```python
from build123d import *

# Parameters (mm, degrees)
F0_R     = 2.5
F1_DEPTH = 7.5
F2_R     = 1
F3_DEPTH = 10
F4_DEPTH = 25


with BuildPart() as f1:
    # F0 (on Top) → F1 (new body)
    with BuildSketch(Plane.XY):
        with BuildLine():
            ThreePointArc((1.4624940646, 33.6666666667), (3.832617517, 34.7501387667), (5.5866740582, 36.6774899598))
            ThreePointArc((5.5866740582, 36.6774899598), (6.2675107251, 38.2771217946), (6.5, 40))
            ThreePointArc((6.5, 40), (-1.7228782054, 46.2675107251), (-5.5866740582, 36.6774899598))
            ThreePointArc((-5.5866740582, 36.6774899598), (-3.832617517, 34.7501387667), (-1.4624940646, 33.6666666667))
            ThreePointArc((-1.4624940646, 33.6666666667), (-0.1677183698, 35.4905940254), (1.5, 34))
            ThreePointArc((1.5, 34), (1.4905940254, 33.8322816302), (1.4624940646, 33.6666666667))
        make_face()
        with Locations((0, 40)):
            Circle(F0_R, mode=Mode.SUBTRACT)
        with BuildLine():
            ThreePointArc((-5.3332565238, 25.44712901), (2.3423382025, 25.8942744974), (9.8131006729, 24.0770233871))
            ThreePointArc((9.8131006729, 24.0770233871), (4.8098794275, 29.40789523), (5.5866740582, 36.6774899598))
            ThreePointArc((5.5866740582, 36.6774899598), (3.832617517, 34.7501387667), (1.4624940646, 33.6666666667))
            ThreePointArc((1.4624940646, 33.6666666667), (0, 32.5), (-1.4624940646, 33.6666666667))
            ThreePointArc((-1.4624940646, 33.6666666667), (-3.832617517, 34.7501387667), (-5.5866740582, 36.6774899598))
            ThreePointArc((-5.5866740582, 36.6774899598), (-4.3898764062, 32.979997265), (-4.9088964418, 29.128452763))
            ThreePointArc((-4.9088964418, 29.128452763), (-4.9503969095, 29.0195498849), (-4.993341291, 28.9112082687))
            Line((-4.993341291, 28.9112082687), (-5.3332565238, 25.44712901))
        make_face()
        with BuildLine():
            ThreePointArc((-10.9419213055, 23.5854692161), (-13.9912480869, -21.9144923959), (26, 0))
            ThreePointArc((26, 0), (21.5770783182, 14.5061949267), (9.8131006729, 24.0770233871))
            ThreePointArc((9.8131006729, 24.0770233871), (2.3423382025, 25.8942744974), (-5.3332565238, 25.44712901))
            Line((-5.3332565238, 25.44712901), (-5.7464520703, 21.2362494006))
            ThreePointArc((-5.7464520703, 21.2362494006), (13.371201413, 17.4702882854), (22, 0))
            ThreePointArc((22, 0), (-10.5068405661, -19.3288980886), (-11.9642092108, 18.4623318668))
            Line((-11.9642092108, 18.4623318668), (-10.9419213055, 23.5854692161))
        make_face()
        with BuildLine():
            ThreePointArc((-9.8131006729, 24.0770233871), (-10.3804210274, 23.837929006), (-10.9419213055, 23.5854692161))
            Line((-10.9419213055, 23.5854692161), (-11.9642092108, 18.4623318668))
            ThreePointArc((-11.9642092108, 18.4623318668), (-9.9487622141, 19.6219807972), (-7.8221766033, 20.5624306245))
            Line((-7.8221766033, 20.5624306245), (-7.3939510007, 24.9264816731))
            ThreePointArc((-7.3939510007, 24.9264816731), (-8.6140032313, 24.5315908235), (-9.8131006729, 24.0770233871))
        make_face()
        with BuildLine():
            ThreePointArc((-7.326121242, 25.6177353666), (-8.504893301, 24.7429137255), (-9.8131006729, 24.0770233871))
            ThreePointArc((-9.8131006729, 24.0770233871), (-8.6140032313, 24.5315908235), (-7.3939510007, 24.9264816731))
            Line((-7.3939510007, 24.9264816731), (-7.326121242, 25.6177353666))
        make_face()
        with BuildLine():
            Line((-9.8358558903, 29.128452763), (-10.9419213055, 23.5854692161))
            ThreePointArc((-10.9419213055, 23.5854692161), (-10.3804210274, 23.837929006), (-9.8131006729, 24.0770233871))
            ThreePointArc((-9.8131006729, 24.0770233871), (-8.504893301, 24.7429137255), (-7.326121242, 25.6177353666))
            Line((-7.326121242, 25.6177353666), (-6.9816296089, 29.128452763))
            Line((-6.9816296089, 29.128452763), (-9.8358558903, 29.128452763))
        make_face()
    extrude(amount=F1_DEPTH)

    # F2 (on face) → F3 (cut)
    with BuildSketch(Plane(origin=(-15.0490291094, 3.0029334363, 0), x_dir=(-0.1956855032, -0.9806667037, 0), z_dir=(-0.9806667037, 0.1956855032, 0))):
        with Locations((-23.4226267785, 3.75)):
            Circle(F2_R)
    extrude(amount=-F3_DEPTH, mode=Mode.SUBTRACT)

    # F2 (on face) → F4 (cut)
    with BuildSketch(Plane(origin=(-15.0490291094, 3.0029334363, 0), x_dir=(-0.1956855032, -0.9806667037, 0), z_dir=(-0.9806667037, 0.1956855032, 0))):
        with BuildLine():
            Line((-20.9883089752, 3.1807049686), (-20.9883089752, 4.3192950314))
            ThreePointArc((-20.9883089752, 4.3192950314), (-25.9226267785, 3.75), (-20.9883089752, 3.1807049686))
        make_face()
        with Locations((-23.4226267785, 3.75)):
            Circle(F2_R, mode=Mode.SUBTRACT)
        with BuildLine():
            ThreePointArc((-20.9883089752, 3.1807049686), (-20.9391016117, 3.4634642327), (-20.9226267785, 3.75))
            ThreePointArc((-20.9226267785, 3.75), (-20.9391016117, 4.0365357673), (-20.9883089752, 4.3192950314))
            Line((-20.9883089752, 4.3192950314), (-20.9883089752, 3.1807049686))
        make_face()
    extrude(amount=F4_DEPTH, mode=Mode.SUBTRACT)


solid = f1.part
```
The listing builds one solid part. Answer for the finished solid, in the listing's coordinates (mm). A direction names the side the tool comes from. Round coordinates to 2 decimals unless told otherwise and drop trailing zeros. Write each loop counter-clockwise with the first axis right and the second up, starting at its lowest first coordinate (ties: lowest second). Pieces come first, ordered by that corner, then holes. Notation, with made-up numbers: (13, 49) -> (41, 49) arc R21 ccw to (41, 70) -> close; hole circle Ø5 at (5.25, 7). An arc over 180 degrees is marked (long way). Answer as a JSON object with one key per item and string values. Group by question number.
Q1. Straight lines are drawn through the part: line 1 along X through (y, z) = (-18.5, 5); line 2 along X through (y, z) = (-1.5, 2.5); line 3 along Y through (x, z) = (-3, 2). For each, find the intervals that lie inside material, in ascending order.
Q2. Which of the six approach directions +Z, -Z, +X, -X, +Y, -Y give full straight-line access (tool end or side, diameter ignored) to faces 1 (the face through (-0.54, 37.56, 3.7)), 2 (the face through (-8, 29.128, 4))?
Q3. Section A-A (z = 1.75) is taken. Write down the section's boundary in (x, y), plus the area to 3 significant figures.
Q4. Each of these flat-tipped pins is pushed along its axis until it touches: pin 1 Ø2 at (x, z) = (-18, 6) entering from -Y; pin 2 Ø1 at (x, z) = (-1.5, 1.5) entering from -Y; pin 3 Ø6.5 at (x, y) = (0, 40) entering from +Z; pin 4 Ø0.9 at (x, z) = (-8, 4) entering from +Y. Where does it stop, or does it pass through?
Q5. Determine the mould class of faces 3 (the face through (4.844, 29.308, 3.698)), 4 (the face through (-8, 21, 7.5)), 5 (the face through (-0.656, 24.03, 3.764)) for opening direction X: pulls with the +X half, pulls with the -X half, needs draft (parallel to the pull), parting line crosses it, or undercut.
Q6. Section B-B (y = -14) is taken. Write down the section's boundary in (x, z), plus the area to 3 significant figures.
Q7. Section C-C (x = -18) is taken. Write down the section's boundary in (y, z).
Check values:
{
 "1": {"line 1": "-18.27 to -11.91, 11.91 to 18.27", "line 2": "-25.96 to -21.95, 21.95 to 25.96", "line 3": "-25.83 to -21.79, 21.79 to 45.77"},
 "2": {"face 1": "+Z, -Z", "face 2": "+Z, -Z, -X, +Y"},
 "3": {"outline": "(-10.94, 23.59) arc R26 ccw (long way) to (9.81, 24.08) arc R8.77 cw to (5.59, 36.68) arc R6.5 ccw (long way) to (-5.59, 36.68) arc R8.77 cw to (-4.99, 28.91) -> (-5.75, 21.24) arc R22 cw (long way) to (-7.82, 20.56) -> (-6.98, 29.13) -> (-9.84, 29.13) -> close; hole circle Ø5 at (0, 40); hole circle Ø3 at (0, 34)", "area": "799 mm^2"},
 "4": {"pin 1": "y = -19.67", "pin 2": "y = -25.98", "pin 3": "z = 7.5", "pin 4": "y = 29.13"},
 "5": {"face 3": "pulls with the +X half", "face 4": "needs draft", "face 5": "undercut"},
 "6": {"outline": "(-21.91, 0) -> (-16.97, 0) -> (-16.97, 7.5) -> (-21.91, 7.5) -> close; (16.97, 0) -> (21.91, 0) -> (21.91, 7.5) -> (16.97, 7.5) -> close", "area": "74.1 mm^2"},
 "7": {"outline": "(-18.76, 0) -> (-12.65, 0) -> (-12.65, 7.5) -> (-18.76, 7.5) -> close; (12.65, 0) -> (18.76, 0) -> (18.76, 7.5) -> (12.65, 7.5) -> close"}
}
